The listing builds one solid part. Answer for the finished solid, in the listing's coordinates (mm). A direction names the side the tool comes from. Round coordinates to 2 decimals unless told otherwise and drop trailing zeros. Order: outer loops, then holes, each group sorted by start corner. A loop starts at its lowest first (then second) coordinate and runs counter-clockwise, first axis right, second up. Notation, with made-up numbers: M 42,-6 L 73,-6 A23 ccw 73,33 Z; hole C 39,45 d6. An arc over 180 degrees is marked long. Put each result on its own line as item: value. Start each with the question number.
1. The part is cut by section D-D (z = -5). Give the vertices of the cut face in (x, y) (3 decimals), then the cut area to 3 significant figures.
2. The part is cut by section C-C (y = 4.5). Give the vertices of the cut face in (x, z) (3 decimals), then the cut area to 3 significant figures.
3. Which of the six approach directions +Z, -Z, +X, -X, +Y, -Y give full straight-line access (tool end or side, diameter ignored) to faces 4 (the face through (12, -29.1, 3)), 5 (the face through (12, 33.1, 3)), 6 (the face through (0, 0, -4)), 7 (the face through (6.35, 1, 5))?
4. Each of these flat-tipped pins is pushed along its axis until it touches: pin 1 Ø4.5 at (x, z) = (14, 7) entering from +Y; pin 2 Ø4 at (y, z) = (-36, 5) entering from +X; pin 3 Ø3 at (y, z) = (20, 2.5) entering from -X. Where does it stop, or does it pass through?
5. The part is cut by section A-A (x = 8). Give the vertices of the cut face in (y, z).
6. The mould has two halves that part along Y. Classify faces 1 (the face through (13.41, -35.565, -13.217)), 2 (the face through (-12, -29.1, 3)), 3 (the face through (10.35, -36, 4)): +Y half, -Y half, draft (parallel to the pull), parting line (faces both ways), or undercut.
7. Consider line 1 (Y direction, x = -12, z = 4); line 2 (X direction, y = -12.5, z = -9) (3 decimals); line 3 (X direction, y = 15.5, z = 5.5). Determine where each line is inside the solid, lowest interval first.
from build123d import *

# Parameters (mm, degrees)
F0_W      = 31.75
F0_H      = 76.2
F1_DEPTH  = 26.81
F2_SIZE   = 5
F3_T      = -4
F4_W      = 4
F4_H      = 10
F5_DEPTH  = 38.1
F7_DEPTH  = 2
F10_DEPTH = 4
F11_SIZE  = 5


# Not quite as in the source:
# - a pattern or mirror of a feature is missing from the dataset's text; its kind, count and spacing are read off the source's solid


with BuildPart() as f1:
    # F0 (on Top) → F1 (new body)
    with BuildSketch(Plane.XY):
        Rectangle(F0_W, F0_H)
    extrude(amount=-F1_DEPTH)

    # F2
    f2_edges = [f1.edges().sort_by_distance(p)[0] for p in [
        (-15.875, -38.1, -13.405),
        (15.875, -38.1, -13.405),
        (-15.875, 38.1, -13.405),
        (15.875, 38.1, -13.405),
    ]]
    chamfer(f2_edges, length=F2_SIZE)

    # F3
    f3_openings = [f1.faces().sort_by_distance(p)[0] for p in [
        (0, 0, -26.81),
    ]]
    offset(amount=F3_T, openings=f3_openings)

    # F4 (on Front) → F5 (join, symmetric)
    with BuildSketch(Plane.XZ):
        with Locations((8.35, 5)):
            Rectangle(F4_W, F4_H)
        with Locations((-8.35, 5)):
            Rectangle(F4_W, F4_H)
    extrude(amount=F5_DEPTH, both=True)

    # F6 (on Front) → F7 (join, symmetric)
    with BuildSketch(Plane.XZ):
        Polygon((-15.875, 0), (-10.35, 0), (-10.35, 10), align=None)
        Polygon((15.875, 0), (10.35, 10), (10.35, 0), align=None)
    f7 = extrude(amount=F7_DEPTH, both=True)

    # F7_copies: F7 across plane
    add(f7.mirror(Plane.ZX.offset(15.55)))

    # F9 (on face) → F10 (join)
    with BuildSketch(Plane.XZ.offset(33.1)):
        Polygon((-10.35, 0), (-10.35, 10), (-15.875, 0), align=None)
        Polygon((10.35, 10), (10.35, 0), (15.875, 0), align=None)
    extrude(amount=-F10_DEPTH)

    # F11
    f11_edges = [f1.edges().sort_by_distance(p)[0] for p in [
        (-8.35, -38.1, 10),
        (8.35, -38.1, 10),
        (-8.35, 38.1, 10),
        (8.35, 38.1, 10),
    ]]
    chamfer(f11_edges, length=F11_SIZE)


solid = f1.part
Resolved:
1. outline: M -15.875,-33.1 L -10.875,-38.1 L 10.875,-38.1 L 15.875,-33.1 L 15.875,33.1 L 10.875,38.1 L -10.875,38.1 L -15.875,33.1 Z; hole M -11.875,-31.443 L -9.218,-34.1 L 9.218,-34.1 L 11.875,-31.443 L 11.875,31.443 L 9.218,34.1 L -9.218,34.1 L -11.875,31.443 Z
1. area: 764 mm2
2. outline: M -15.875,-26.81 L -11.875,-26.81 L -11.875,-4 L 11.875,-4 L 11.875,-26.81 L 15.875,-26.81 L 15.875,0 L 10.35,0 L 10.35,10 L 6.35,10 L 6.35,0 L -6.35,0 L -6.35,10 L -10.35,10 L -10.35,0 L -15.875,0 Z
2. area: 389 mm2
3. face 4: +Z, +X
3. face 5: +Z, +X, +Y
3. face 6: -Z
3. face 7: +Z, +Y, -Y
4. pin 1: y = 33.1
4. pin 2: x = 10.35
4. pin 3: x = -10.35
5. outline: M -38.1,-26.81 L -34.1,-26.81 L -34.1,-4 L 34.1,-4 L 34.1,-26.81 L 38.1,-26.81 L 38.1,5 L 33.1,10 L -33.1,10 L -38.1,5 Z
6. face 1: -Y half
6. face 2: undercut
6. face 3: draft
7. line 1: -33.1 to -29.1, -2 to 2, 29.1 to 33.1
7. line 2: -15.875 to -11.875, 11.875 to 15.875
7. line 3: -10.35 to -6.35, 6.35 to 10.35
